Read the model definition and answer for the solid it produces. Units are mm, in the model's axes. A direction names the side the tool comes from. Give positions to 0.01 mm unless a question says otherwise; leave off trailing zeros. Loops run counter-clockwise (first coordinate to the right, second up) from the corner with the lowest first, then second, coordinate; pieces in that order, holes last. Notation, with made-up numbers: M 42,-32 L 91,-32 A35 ccw 91,5 Z; hole C -29,31.25 d7. An arc over 180 degrees is marked long. Return JSON: item names as keys, results as strings. Group by question number.
```python
from build123d import *

# Parameters (mm, degrees)
SKETCH1_R           = 27
BOSS_EXTRUDE2_DEPTH = 3
SKETCH3_W           = 11
SKETCH3_H           = 11
CUT_EXTRUDE1_DEPTH  = 3
SKETCH5_W           = 12
SKETCH5_H           = 12
SKETCH5_W_2         = 11
SKETCH5_H_2         = 11
BOSS_EXTRUDE3_DEPTH = 60
SKETCH6_W           = 8
SKETCH6_H           = 50
CUT_EXTRUDE2_DEPTH  = 60


with BuildPart() as part:
    # Sketch1 → Boss-Extrude2 (new body)
    with BuildSketch(Plane(origin=(0, 0, 0), x_dir=(1, 0, 0), z_dir=(0, 1, 0))):
        with Locations(Location((0, 0, 0), (0, 0, 270))):
            Circle(SKETCH1_R)
    extrude(amount=BOSS_EXTRUDE2_DEPTH)

    # Sketch3 → Cut-Extrude1 (cut)
    with BuildSketch(Plane(origin=(0, 3, 0), x_dir=(1, 0, 0), z_dir=(0, 1, 0))):
        with Locations((16.527901815, 0.208370768)):
            Rectangle(SKETCH3_W, SKETCH3_H)
    extrude(amount=-CUT_EXTRUDE1_DEPTH, mode=Mode.SUBTRACT)

    # Sketch5 → Boss-Extrude3 (add)
    with BuildSketch(Plane(origin=(0, 3, 0), x_dir=(1, 0, 0), z_dir=(0, 1, 0))):
        with Locations((16.527901815, 0.208370768)):
            Rectangle(SKETCH5_W, SKETCH5_H)
        with Locations((16.527901815, 0.208370768)):
            Rectangle(SKETCH5_W_2, SKETCH5_H_2, mode=Mode.SUBTRACT)
    extrude(amount=BOSS_EXTRUDE3_DEPTH)

    # Sketch6 → Cut-Extrude2 (cut)
    with BuildSketch(Plane(origin=(22.527901815, 0, 0), x_dir=(0, 0, -1), z_dir=(1, 0, 0))):
        with Locations((0.208370768, 33)):
            Rectangle(SKETCH6_W, SKETCH6_H)
    extrude(amount=-CUT_EXTRUDE2_DEPTH, mode=Mode.SUBTRACT)


solid = part.part
```
1. The mould has two halves that part along Z. Classify faces 5 (the flat face through (0, 3, 0)), 6 (the flat face through (16, 33, -6.208)), 7 (the flat face through (22.028, 31, 5)): +Z half, -Z half, draft (parallel to the pull), parting line (faces both ways), or undercut.
2. Straight lines are drawn through the part: line 1 along Z through (x, y) = (13.5, 34.5); line 2 along X through (y, z) = (33, -5); line 3 along Y through (x, z) = (-20, 3.5). For each, find the intervals that lie inside material, in ascending order.
3. Find section D-D (z = 12). Write down the section's boundary in (x, y).
4. Find section C-C (z = 0). Write down the section's boundary in (x, y).
5. Find section B-B (x = 20). Write down the section's boundary in (y, z), and give its area (3 significant figures).
6. Flat-ended cylindrical pins translate along their axes: P1, Ø9, axis at y = 33.5, z = 0, coming from the -X side; P2, Ø13, axis at x = 18.5, y = 37, coming from the -Z side; P3, Ø9.5, axis at y = 36, z = 2, coming from the +X side; P4, Ø6, axis at y = 25, z = -1, coming from the -X side. Find the tip coordinate at first contact, or state that the pin passes through.
7. Find section A-A (y = 38). Write down the section's boundary in (x, z), and give its area (3 significant figures).
8. For faces 1 (the flat face through (10.528, 33, 4)), 2 (the flat face through (22.528, 33, 4)), 3 (the flat face through (16, 31, 5.292)), 4 (the flat face through (16, 33, 5.792)), determine the directions among +Z, -Z, +X, -X, +Y, -Y from which every point of the face is accessible in a straight line to the end or side of a thin tool.
Result:
{
 "1": {"face 5": "draft", "face 6": "-Z half", "face 7": "undercut"},
 "2": {"line 1": "z = -6.21 to -5.71, 5.29 to 5.79", "line 2": "x = 10.53 to 11.03, 22.03 to 22.53", "line 3": "y = 0 to 3"},
 "3": {"outline": "M -24.19,0 L 24.19,0 L 24.19,3 L -24.19,3 Z"},
 "4": {"outline": "M -27,0 L 11.03,0 L 11.03,8 L 10.53,8 L 10.53,3 L -27,3 Z; M 10.53,58 L 11.03,58 L 11.03,63 L 10.53,63 Z; M 22.03,0 L 27,0 L 27,3 L 22.53,3 L 22.53,8 L 22.03,8 Z; M 22.03,58 L 22.53,58 L 22.53,63 L 22.03,63 Z"},
 "5": {"outline": "M 0,-18.14 L 3,-18.14 L 3,-6.21 L 63,-6.21 L 63,-5.71 L 0,-5.71 Z; M 0,5.29 L 63,5.29 L 63,5.79 L 3,5.79 L 3,18.14 L 0,18.14 Z", "area": "136 mm2"},
 "6": {"P1": "stops at x = 10.53", "P2": "stops at z = -6.21", "P3": "stops at x = 22.53", "P4": "passes through"},
 "7": {"outline": "M 10.53,-6.21 L 22.53,-6.21 L 22.53,-4.21 L 22.03,-4.21 L 22.03,-5.71 L 11.03,-5.71 L 11.03,-4.21 L 10.53,-4.21 Z; M 10.53,3.79 L 11.03,3.79 L 11.03,5.29 L 22.03,5.29 L 22.03,3.79 L 22.53,3.79 L 22.53,5.79 L 10.53,5.79 Z", "area": "15.0 mm2"},
 "8": {"face 1": "+Z, -Z, -X, +Y", "face 2": "+Z, -Z, +X, +Y", "face 3": "+Y, -Y", "face 4": "+Z, +X, -X, +Y"}
}
